Read the model definition and answer for the solid it produces. Units are mm, in the model's axes. Coordinates: 2 decimals unless noted, no trailing zeros. Loops run counter-clockwise (first coordinate to the right, second up) from the corner with the lowest first, then second, coordinate; pieces in that order, holes last.
from build123d import *

# Parameters (mm, degrees)
SKETCH_1_W          = 15
SKETCH_1_H          = 10
SKETCH_1_W_2        = 13
SKETCH_1_H_2        = 8
EXTRUDE_1_DEPTH     = 125
SKETCH_2_R          = 2.1
CUT_EXTRUDE_1_DEPTH = 127.293309403
SKETCH_3_R          = 1.6
CUT_EXTRUDE_2_DEPTH = 127.293309403


with BuildPart() as part:
    # 草图1 → 拉伸-薄壁1 (new body)
    with BuildSketch(Plane.XY):
        with Locations((7.5, -5)):
            Rectangle(SKETCH_1_W, SKETCH_1_H)
        with Locations((7.5, -5)):
            Rectangle(SKETCH_1_W_2, SKETCH_1_H_2, mode=Mode.SUBTRACT)
    extrude(amount=EXTRUDE_1_DEPTH)

    # 草图2 → 切除-拉伸1 (cut, through all)
    with BuildSketch(Plane(origin=(15, 0, 0), x_dir=(0, 0, -1), z_dir=(1, 0, 0))):
        with Locations(Location((-120, -5, 0), (0, 0, 90))):
            Circle(SKETCH_2_R)
        with Locations(Location((-110, -5, 0), (0, 0, 270))):
            Circle(SKETCH_2_R)
        with Locations(Location((-15, -5, 0), (0, 0, 90))):
            Circle(SKETCH_2_R)
        with Locations(Location((-5, -5, 0), (0, 0, 270))):
            Circle(SKETCH_2_R)
    extrude(amount=-CUT_EXTRUDE_1_DEPTH, mode=Mode.SUBTRACT)

    # 草图3 → 切除-拉伸2 (cut, through all)
    with BuildSketch(Plane.XZ.offset(10)):
        with Locations(Location((3.75, 67.5, 0), (0, 0, 270))):
            Circle(SKETCH_3_R)
        with Locations(Location((11.25, 67.5, 0), (0, 0, 270))):
            Circle(SKETCH_3_R)
        with Locations(Location((11.25, 57.5, 0), (0, 0, 270))):
            Circle(SKETCH_3_R)
        with Locations(Location((3.75, 57.5, 0), (0, 0, 270))):
            Circle(SKETCH_3_R)
        with Locations(Location((3.75, 120, 0), (0, 0, 270))):
            Circle(SKETCH_3_R)
        with Locations(Location((11.25, 120, 0), (0, 0, 270))):
            Circle(SKETCH_3_R)
        with Locations(Location((11.25, 110, 0), (0, 0, 270))):
            Circle(SKETCH_3_R)
        with Locations(Location((3.75, 110, 0), (0, 0, 270))):
            Circle(SKETCH_3_R)
        with Locations(Location((3.75, 15, 0), (0, 0, 270))):
            Circle(SKETCH_3_R)
        with Locations(Location((11.25, 15, 0), (0, 0, 270))):
            Circle(SKETCH_3_R)
        with Locations(Location((11.25, 5, 0), (0, 0, 270))):
            Circle(SKETCH_3_R)
        with Locations(Location((3.75, 5, 0), (0, 0, 270))):
            Circle(SKETCH_3_R)
    extrude(amount=-CUT_EXTRUDE_2_DEPTH, mode=Mode.SUBTRACT)


solid = part.part
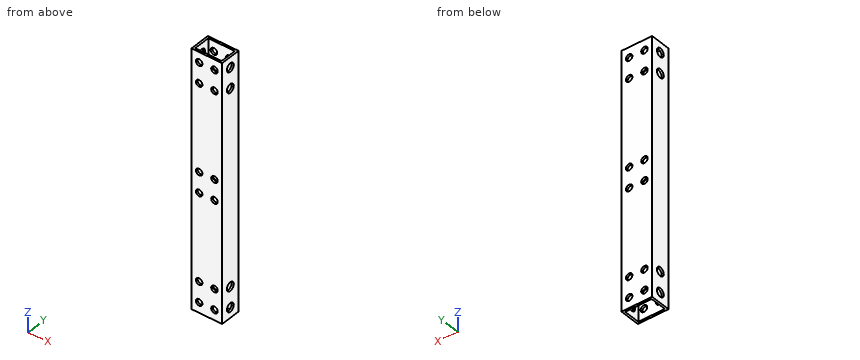
Item 1: A cutting plane is placed at C-C on x = 7. Determine the outline of the cut face in (y, z).
Numbers:
outline: (-10, 0) - (-9, 0) - (-9, 125) - (-10, 125) - close; (-1, 0) - (0, 0) - (0, 125) - (-1, 125) - close
Item 2: Find the intervals of material crossed by line 1 along Z through (x, y) = (14.45, -5); line 2 along X through (y, z) = (-9.75, 15); line 3 along Y through (x, z) = (6.5, 108), in increasing order.
Numbers:
line 1: z = 0 to 2.9, 7.1 to 12.9, 17.1 to 107.9, 112.1 to 117.9, 122.1 to 125
line 2: x = 0 to 2.15, 5.35 to 9.65, 12.85 to 15
line 3: y = -10 to -9, -1 to 0
Item 3: A cutting plane is placed at B-B on z = 57.5. Determine the outline of the cut face in (x, y).
Numbers:
outline: (0, -10) - (2.15, -10) - (2.15, -9) - (1, -9) - (1, -1) - (2.15, -1) - (2.15, 0) - (0, 0) - close; (5.35, -10) - (9.65, -10) - (9.65, -9) - (5.35, -9) - close; (5.35, -1) - (9.65, -1) - (9.65, 0) - (5.35, 0) - close; (12.85, -10) - (15, -10) - (15, 0) - (12.85, 0) - (12.85, -1) - (14, -1) - (14, -9) - (12.85, -9) - close
Item 4: A cutting plane is placed at A-A on z = 110. Give the number of separate pieces and of enclosed holes in the cut face, then the cut area to 3 significant figures.
Numbers:
separate pieces: 6
enclosed holes: 0
area: 24.8 mm2
Item 5: Given pin 1 (5 mm diameter, centred on x = 3.75, z = 110, fed in from -Y); pin 2 (3 mm diameter, centred on x = 3.75, z = 120, fed in from -Y), each flat-ended and moving along its own axis, determine where each tip first touches the part or whether it passes through.
Numbers:
pin 1: stops at y = -10
pin 2: passes through
Item 6: A cutting plane is placed at D-D on z = 41. Determine the outline of the cut face in (x, y), then the cut area to 3 significant figures.
Numbers:
outline: (0, -10) - (15, -10) - (15, 0) - (0, 0) - close; hole (1, -9) - (14, -9) - (14, -1) - (1, -1) - close
area: 46.0 mm2
